Verification items for the finished model (mm, model axes). Face numbers are marked on the shaded views. A direction names the side the tool comes from. Coordinates: 2 decimals unless noted, no trailing zeros. Write each loop counter-clockwise with the first axis right and the second up, starting at its lowest first coordinate (ties: lowest second). Pieces come first, ordered by that corner, then holes. Notation, with made-up numbers: (61, 51) - (110, 51) arc R19 ccw to (110, 88) - close; hole circle Ø11 at (-32, 42.5). An arc over 180 degrees is marked (long way). Use CSV: the item, a comma, the result in double quotes. Start each with the question number.
```python
from build123d import *

# Parameters (mm, degrees)
SALIENTE_EXTRUIR1_DEPTH = 40
REDONDEO1_RADIUS        = 20
REDONDEO1_LENGTH        = 18
CROQUIS3_W              = 25.4
CROQUIS3_H              = 25.4
CORTAR_EXTRUIR2_DEPTH   = 65
CROQUIS4_R              = 3.96875
CORTAR_EXTRUIR3_DEPTH   = 292.21181988
REDONDEO3_R             = 6.35


with BuildPart() as part:
    # Croquis1 → Saliente-Extruir1 (new body)
    with BuildSketch(Plane(origin=(0, 0, 0), x_dir=(1, 0, 0), z_dir=(0, 1, 0))):
        Polygon((283.9431, 16.4), (283.9431, -34.4), (215, -34.4), (200, -19.4), (200, -18), (0, -18), (0, 0), (200, 0), (200, 1.4), (215, 16.4), align=None)
    extrude(amount=SALIENTE_EXTRUIR1_DEPTH)

    # Redondeo1: full round fillet: the end face becomes a half cylinder, R = half its width
    redondeo1_face = Plane((0, 20, 9), x_dir=(0, 0, 1), z_dir=(-1, 0, 0))  # on the end face: x along it, z out of the body
    redondeo1_slab = redondeo1_face.offset(-REDONDEO1_RADIUS / 2) * Box(REDONDEO1_LENGTH, 2 * REDONDEO1_RADIUS, REDONDEO1_RADIUS, mode=Mode.PRIVATE)  # the body's end, R deep
    redondeo1_round = Plane((20, 20, 9), x_dir=(-1, 0, 0), z_dir=(0, 0, 1)) * Cylinder(REDONDEO1_RADIUS, REDONDEO1_LENGTH, mode=Mode.PRIVATE)  # its axis R under the face
    add(redondeo1_slab - redondeo1_round, mode=Mode.SUBTRACT)

    # Croquis3 → Cortar-Extruir2 (cut)
    with BuildSketch(Plane(origin=(283.9431, 0, 0), x_dir=(0, 0, -1), z_dir=(1, 0, 0))):
        with Locations((-9, 20)):
            Rectangle(CROQUIS3_W, CROQUIS3_H)
    extrude(amount=-CORTAR_EXTRUIR2_DEPTH, mode=Mode.SUBTRACT)

    # Croquis4 → Cortar-Extruir3 (cut, through all)
    with BuildSketch(Plane.XY.offset(34.4)):
        with Locations((266.4431, 20)):
            Circle(CROQUIS4_R)
        with Locations((236.4431, 20)):
            Circle(CROQUIS4_R)
    extrude(amount=-CORTAR_EXTRUIR3_DEPTH, mode=Mode.SUBTRACT)

    # Redondeo3
    redondeo3_edges = [part.edges().sort_by_distance(p)[0] for p in [
        (251.4431, 7.3, 21.7),
        (251.4431, 32.7, 21.7),
        (251.4431, 32.7, -3.7),
        (251.4431, 7.3, -3.7),
    ]]
    fillet(redondeo3_edges, radius=REDONDEO3_R)


solid = part.part
```
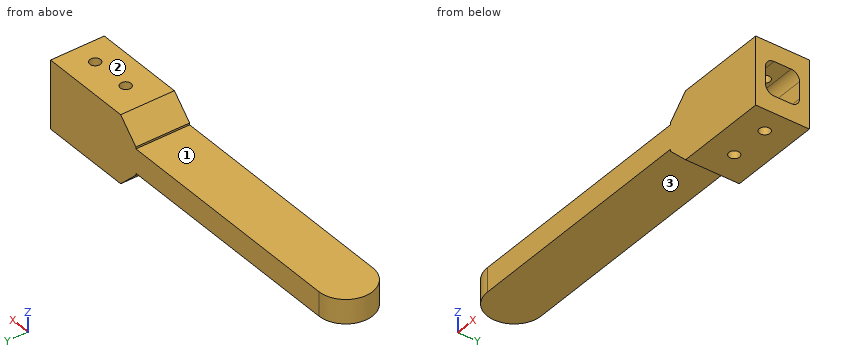
Q1. Cross-section at B-B (y = 20). State how many separate pieces and enclosed holes the cut face has, plus the area to 3 significant figures.
Q2. Gauge pin test, flat ends, axial feed: pin 1 (1.5 mm diameter, centred on x = 40.5, y = 35, fed in from -Z); pin 2 (0.7 mm diameter, centred on y = 11.5, z = -0.5, fed in from -X); pin 3 (12 mm diameter, centred on x = 111, y = 13.5, fed in from +Z). Record the tip position at first contact, or that the pin passes through.
Q3. Cross-section at D-D (y = 3.5). Record the cut outline in (x, z), plus the area to 3 significant figures.
Q4. Scan lines: line 1 along X through (y, z) = (19, -8.5); line 2 along Z through (x, y) = (221.5, 24.5); line 3 along Z through (x, y) = (45.5, 13.5). Record each from-to range of solid material in increasing order. Write a range as from..to.
Q5. Tool access check on the marked faces 1, 2 and 3. Record the directions out of +Z, -Z, +X, -X, +Y, -Y that give a thin tool (end or side, any length) a straight path to the whole face; none if there is none.
Q6. Cross-section at C-C (z = -9). Record the cut outline in (x, y).
Q7. Cross-section at A-A (x = 245). Record the cut outline in (y, z).
Reply:
1,separate pieces,"5"
1,enclosed holes,"0"
1,area,"5,590 mm^2"
2,pin 1,"z = 0"
2,pin 2,"x = 200"
2,pin 3,"z = 18"
3,outline,"(8.7, 0) - (200, 0) - (200, -1.4) - (215, -16.4) - (283.94, -16.4) - (283.94, 34.4) - (215, 34.4) - (200, 19.4) - (200, 18) - (8.7, 18) - close"
3,area,"7,480 mm^2"
4,line 1,"207.1..232.6, 240.28..262.6, 270.28..283.94"
4,line 2,"-16.4..-3.7, 21.7..34.4"
4,line 3,"0..18"
5,face 1,"+Z, -X, +Y, -Y"
5,face 2,"+Z, +X, -X, +Y, -Y"
5,face 3,"-Z, -X, +Y, -Y"
6,outline,"(207.6, 0) - (283.94, 0) - (283.94, 40) - (207.6, 40) - close; hole circle Ø7.94 at (236.44, 20); hole circle Ø7.94 at (266.44, 20)"
7,outline,"(0, -16.4) - (40, -16.4) - (40, 34.4) - (0, 34.4) - close; hole (7.3, 2.65) arc R6.35 ccw to (13.65, -3.7) - (26.35, -3.7) arc R6.35 ccw to (32.7, 2.65) - (32.7, 15.35) arc R6.35 ccw to (26.35, 21.7) - (13.65, 21.7) arc R6.35 ccw to (7.3, 15.35) - close"
